```python
from build123d import *

# Parameters (mm, degrees)
F0_R     = 3.175
F0_R_2   = 5.55625
F1_DEPTH = 6.35


with BuildPart() as f1:
    # F0 (on Front) → F1 (new body)
    with BuildSketch(Plane.XZ):
        Polygon((38.1, -57.15), (38.1, 57.15), (12.7, 57.15), (-38.1, -31.75), (-38.1, -57.15), align=None)
        with Locations((-25.4, -44.45)):
            Circle(F0_R, mode=Mode.SUBTRACT)
        with Locations((0, -44.45)):
            Circle(F0_R, mode=Mode.SUBTRACT)
        with Locations((25.4, -44.45)):
            Circle(F0_R, mode=Mode.SUBTRACT)
        with Locations((25.4, -19.05)):
            Circle(F0_R_2, mode=Mode.SUBTRACT)
        with Locations((25.4, 6.35)):
            Circle(F0_R_2, mode=Mode.SUBTRACT)
        with Locations((25.4, 25.4)):
            Circle(F0_R_2, mode=Mode.SUBTRACT)
        with Locations((25.4, 44.45)):
            Circle(F0_R_2, mode=Mode.SUBTRACT)
    extrude(amount=F1_DEPTH)


solid = f1.part
```
Part model, mm, in its own coordinate system. Round coordinates to 2 decimals unless told otherwise and drop trailing zeros. Loops run counter-clockwise (first coordinate to the right, second up) from the corner with the lowest first, then second, coordinate; pieces in that order, holes last.
Item 1: Drop flat-ended pins along their axis: P1, Ø10, axis at x = -25.4, z = -44.45, coming from the -Y side; P2, Ø10, axis at x = 25.4, z = 6.35, coming from the -Y side; P3, Ø1.5, axis at x = -7, y = -4, coming from the +Z side. Give the stop position or say it passes through.
Item 2: Cut at B-B, the plane x = 25.4. Give the cut face in (y, z) (3 decimals), then the cut area to 3 significant figures.
Item 3: Cut at A-A, the plane z = -44.45. Give the cut face in (x, y) (3 decimals).
Item 4: Cut at C-C, the plane y = -5. State how many separate pieces and enclosed holes the cut face has, then the cut area to 3 significant figures.
Item 5: Cut at D-D, the plane x = 1.5. Give the cut face in (y, z).
Item 6: Mould opens along Z. For faces 1 (the face through (8, 0, -12)), 2 (the face through (-1, -3, -57.15)), 3 (the face through (27.107, -3.131, -41.773)), 4 (the face through (26, -3, 57.15)) say: +Z half, -Z half, draft (parallel to the pull), parting line (faces both ways), or undercut.
Item 7: Drill centre lines: line 1 (Z direction, x = 25.4, y = -4.25) (3 decimals); line 2 (Z direction, x = 0, y = -3) (3 decimals); line 3 (Z direction, x = -25.4, y = -1.25) (3 decimals). Where is each one in solid material? Low to high.
A:
1. P1: stops at y = -6.35
1. P2: passes through
1. P3: stops at z = 23.99
2. outline: (-6.35, -57.15) - (0, -57.15) - (0, -47.625) - (-6.35, -47.625) - close; (-6.35, -41.275) - (0, -41.275) - (0, -24.606) - (-6.35, -24.606) - close; (-6.35, -13.494) - (0, -13.494) - (0, 0.794) - (-6.35, 0.794) - close; (-6.35, 11.906) - (0, 11.906) - (0, 19.844) - (-6.35, 19.844) - close; (-6.35, 30.956) - (0, 30.956) - (0, 38.894) - (-6.35, 38.894) - close; (-6.35, 50.006) - (0, 50.006) - (0, 57.15) - (-6.35, 57.15) - close
2. area: 403 mm2
3. outline: (-38.1, -6.35) - (-28.575, -6.35) - (-28.575, 0) - (-38.1, 0) - close; (-22.225, -6.35) - (-3.175, -6.35) - (-3.175, 0) - (-22.225, 0) - close; (3.175, -6.35) - (22.225, -6.35) - (22.225, 0) - (3.175, 0) - close; (28.575, -6.35) - (38.1, -6.35) - (38.1, 0) - (28.575, 0) - close
4. separate pieces: 1
4. enclosed holes: 7
4. area: 5,970 mm2
5. outline: (-6.35, -57.15) - (0, -57.15) - (0, -47.25) - (-6.35, -47.25) - close; (-6.35, -41.65) - (0, -41.65) - (0, 37.55) - (-6.35, 37.55) - close
6. face 1: draft
6. face 2: -Z half
6. face 3: undercut
6. face 4: +Z half
7. line 1: z = -57.15 to -47.625, -41.275 to -24.606, -13.494 to 0.794, 11.906 to 19.844, 30.956 to 38.894, 50.006 to 57.15
7. line 2: z = -57.15 to -47.625, -41.275 to 34.925
7. line 3: z = -57.15 to -47.625, -41.275 to -9.525
